The drawing under review shows one solid part. Ordinate dimensions are in mm from its lowest x, y, z. Give positions to 0.01 mm unless a question says otherwise; leave off trailing zeros. Order: outer loops, then holes, each group sorted by start corner. A loop starts at its lowest first (then second) coordinate and runs counter-clockwise, first axis right, second up. Notation, with made-up numbers: (-29.5, 88) -> (11.5, 88) arc R15 cw to (11.5, 104) -> close; hole circle Ø3 at (46.5, 52). An arc over 180 degrees is marked (long way). Use CSV: the item, a comma, the result in double quotes. Start each with the question number.
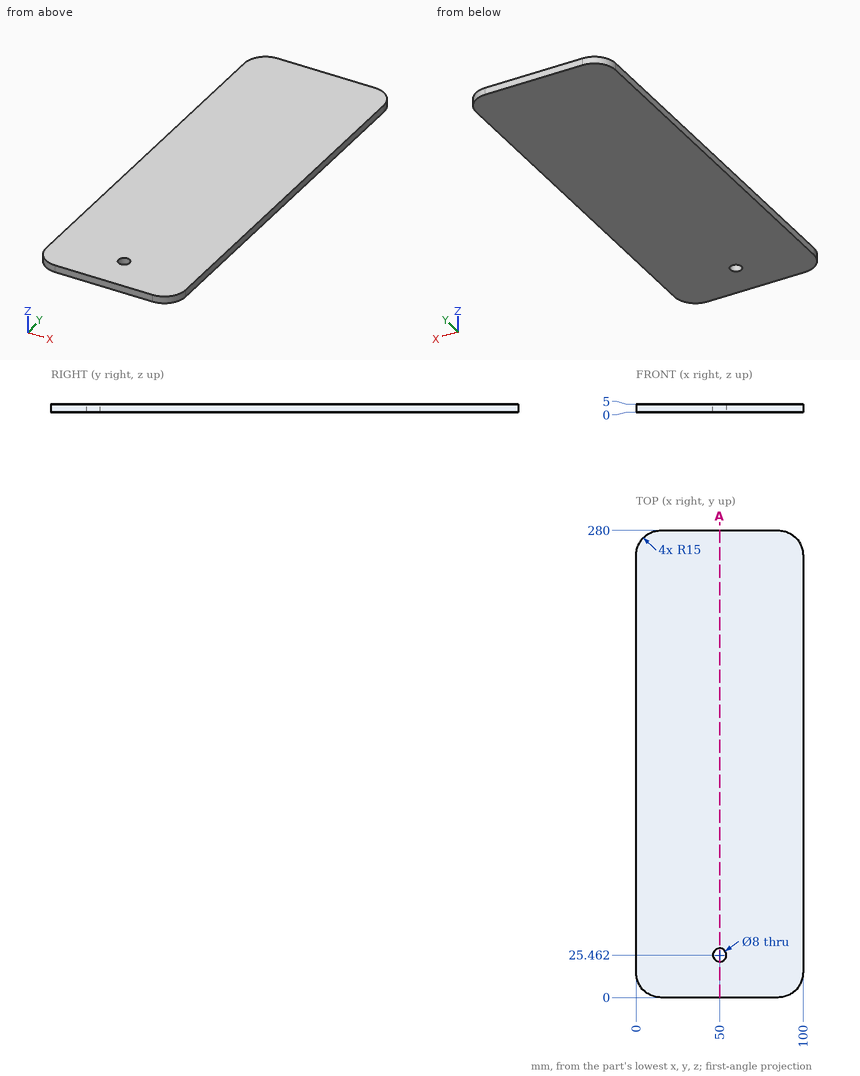
1. To check wall thickness, follow L1, parallel to Y at x = 50, z = 3.45; L2, parallel to Y at x = 51.5, z = 4.3 (1 decimal); L3, parallel to Y at x = 87, z = 0.8. State the ranges of each line that lie inside material, in increasing order. Write a range as [from, to].
2. Clearance check with a flat-ended pin moving along its axis: P1, Ø1, axis at x = 11, z = 3, coming from the -Y side. State where the tip first meets the part, or that it passes through.
3. Consider section A-A (x = 50). State the section outline as (y, z) points.
Answer list:
1,L1,"[0, 21.46], [29.46, 280]"
1,L2,"[0, 21.8], [29.2, 280]"
1,L3,"[0.13, 279.87]"
2,P1,"y = 0.41"
3,outline,"(0, 0) -> (21.46, 0) -> (21.46, 5) -> (0, 5) -> close; (29.46, 0) -> (280, 0) -> (280, 5) -> (29.46, 5) -> close"
